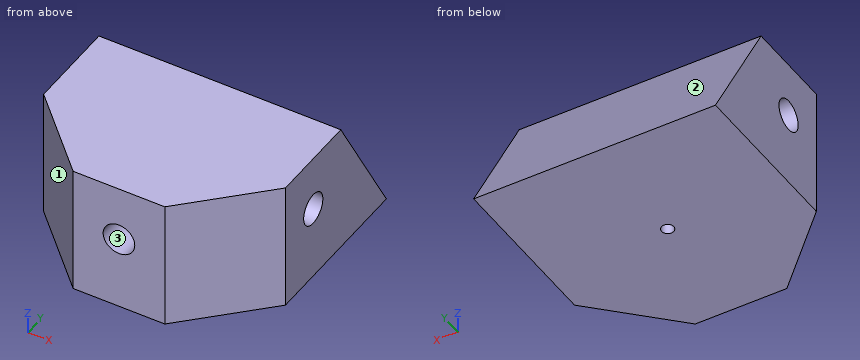
```python
from build123d import *

# Parameters (mm, degrees)
SKETCH2_W               = 330.2
SKETCH2_H               = 330.2
BOSS_EXTRUDE1_DEPTH     = 177.8
CUT_EXTRUDE1_DEPTH      = 410.759551445
CUT_EXTRUDE1_DEPTH_BACK = 410.759551445
SKETCH3_R               = 21.59
SKETCH5_R               = 8.382
CUT_EXTRUDE3_DEPTH      = 101.6
SKETCH6_R               = 21.59
CUT_EXTRUDE4_DEPTH      = 165.1
CHAMFER6_SIZE           = 103.195588962
CHAMFER6_SIZE_2         = 178.7400032
CHAMFER7_SIZE           = 102.5400032


with BuildPart() as part:
    # Sketch2 → Boss-Extrude1 (new body)
    with BuildSketch(Plane.XY):
        Rectangle(SKETCH2_W, SKETCH2_H)
    extrude(amount=BOSS_EXTRUDE1_DEPTH)

    # Sketch3 → Cut-Extrude1 (cut, two sides: drawn at the far end of the back side and taken through both)
    with BuildSketch(Plane(origin=(165.1, 0, 0), x_dir=(0, 0, -1), z_dir=(1, 0, 0)).offset(-CUT_EXTRUDE1_DEPTH_BACK)):
        with Locations((-101.6, 0)):
            Circle(SKETCH3_R)
    extrude(amount=CUT_EXTRUDE1_DEPTH + CUT_EXTRUDE1_DEPTH_BACK, mode=Mode.SUBTRACT)

    # Sketch5 → Cut-Extrude3 (cut)
    with BuildSketch(Plane(origin=(0, 0, 0), x_dir=(-1, 0, 0), z_dir=(0, 0, -1))):
        Circle(SKETCH5_R)
    extrude(amount=-CUT_EXTRUDE3_DEPTH, mode=Mode.SUBTRACT)

    # Sketch6 → Cut-Extrude4 (cut)
    with BuildSketch(Plane.XZ.offset(165.1)):
        with Locations(Location((0, 101.6, 0), (0, 0, 270))):
            Circle(SKETCH6_R)
    extrude(amount=-CUT_EXTRUDE4_DEPTH, mode=Mode.SUBTRACT)

    # Chamfer6
    # the kernel refuses this chamfer: 178.7400032, 103.195588962 mm, written as the material it takes off along each edge
    with BuildSketch(Plane(origin=(627.515716064, 165.1, 177.8), x_dir=(0, -1, 0), z_dir=(-1, 0, 0))) as chamfer6_piece_1:
        Polygon((CHAMFER6_SIZE, 0), (0, -CHAMFER6_SIZE_2), (0, 0), align=None)
    extrude(amount=1255.031432128, mode=Mode.SUBTRACT)

    # Chamfer7
    chamfer7_edges = [part.edges().sort_by_distance(p)[0] for p in [
        (165.1, -165.1, 88.9),
        (-165.1, -165.1, 88.9),
    ]]
    chamfer(chamfer7_edges, length=CHAMFER7_SIZE)


solid = part.part
```
Read the model definition and answer for the solid it produces. Units are mm, in the model's axes. Face numbers are marked on the shaded views. Give positions to 0.01 mm unless a question says otherwise; leave off trailing zeros. Write each loop counter-clockwise with the first axis right and the second up, starting at its lowest first coordinate (ties: lowest second). Pieces come first, ordered by that corner, then holes. Notation, with made-up numbers: M 36,73.5 L 69,73.5 A31 cw 69,101.5 Z; hole C 71,15.5 d4. An arc over 180 degrees is marked long. Put each result on its own line as item: value. Start each with the question number.
1. The part is cut by section C-C, the plane z = 101.6. Give the vertices of the cut face in (x, y), and give its area (3 significant figures).
2. For a pull along Z with two mould halves and no side action, classify the marked faces 1, 2 and 3 as released by +Z, released by -Z, zero draft, split by the parting line, or undercut.
3. The part is cut by section A-A, the plane x = 117. Give the vertices of the cut face in (y, z).
4. Consider line 1 along X through (y, z) = (0, 55); line 2 along Z through (x, y) = (91, 0); line 3 along Z through (x, y) = (-10.5, -37). Determine where each line is inside the solid, lowest interval first.
5. The part is cut by section B-B, the plane y = -125. Give the vertices of the cut face in (x, z).
6. The part is cut by section D-D, the plane z = 42.5. Give the vertices of the cut face in (x, y).
7. Each of these flat-tipped pins is pushed along its axis until it touches: pin 1 Ø1 at (x, y) = (-24.5, -36.5) entering from -Z; pin 2 Ø5 at (x, z) = (7.5, 85.5) entering from +Y; pin 3 Ø6 at (x, z) = (-108, 123) entering from -Y; pin 4 Ø1.5 at (y, z) = (-80, 151) entering from -X. Where does it stop, or does it pass through?
Final values:
1. outline: M -165.1,-62.56 L -62.56,-165.1 L -21.59,-165.1 L -21.59,-21.59 L -165.1,-21.59 Z; M -165.1,21.59 L 165.1,21.59 L 165.1,105.9 L -165.1,105.9 Z; M 21.59,-165.1 L 62.56,-165.1 L 165.1,-62.56 L 165.1,-21.59 L 21.59,-21.59 Z
1. area: 58,500 mm²
2. face 1: zero draft
2. face 2: released by +Z
2. face 3: undercut
3. outline: M -110.66,0 L 164.56,0 L 61.9,177.8 L -110.66,177.8 Z; hole C 0,101.6 d43.18
4. line 1: x = -165.1 to -8.38, 8.38 to 165.1
4. line 2: z = 0 to 80.01, 123.19 to 177.8
4. line 3: z = 0 to 82.74, 120.46 to 177.8
5. outline: M -102.66,0 L 102.66,0 L 102.66,177.8 L -102.66,177.8 Z; hole C 0,101.6 d43.18
6. outline: M -165.1,-62.56 L -62.56,-165.1 L 62.56,-165.1 L 165.1,-62.56 L 165.1,140.02 L -165.1,140.02 Z; hole C 0,0 d16.76
7. pin 1: stops at z = 0
7. pin 2: stops at y = 116.64
7. pin 3: stops at y = -122.66
7. pin 4: stops at x = -148.41
